CAD build for the part. Positions are in the model's coordinates, mm. Round coordinates to 2 decimals unless told otherwise and drop trailing zeros. Order: outer loops, then holes, each group sorted by start corner. A loop starts at its lowest first (then second) coordinate and runs counter-clockwise, first axis right, second up. Notation, with made-up numbers: (17, 74.5) -> (39, 74.5) arc R19 ccw to (39, 93.5) -> close; hole circle Ø2 at (83.25, 20). An arc over 180 degrees is marked (long way). Return JSON: item names as keys, results as strings. Group by question number.
Q1. Cut at C-C (y = -5). Count the separate pieces of the cut face and the enclosed holes in it, then the cut area to 3 significant figures.
Q2. Cut at A-A (x = 138). Write the cut outline in (y, z).
Q3. Probe line 1 along Z through (x, y) = (354.5, -9.5); line 2 along Z through (x, y) = (149.5, -2.25); line 3 along Z through (x, y) = (480.5, -7.25). List the from-to ranges inside material, lowest first.
Q4. Cut at B-B (z = 173.5). Write the cut outline in (x, y), then the cut area to 3 significant figures.
Q5. Flat gauge pins, fed straight in: pin 1 (5 mm diameter, centred on y = -9, z = 80.5, fed in from +X); pin 2 (5 mm diameter, centred on x = 439, y = -6.5, fed in from +Z). Where does each tip first touch, or does it go through?
Q6. Cut at D-D (x = 213.5). Write the cut outline in (y, z).
from build123d import *

# Parameters (mm, degrees)
PAD_DEPTH       = 10
SKETCH001_W     = 379
SKETCH001_H     = 305
SKETCH001_W_2   = 413
SKETCH001_H_2   = 45
POCKET_DEPTH    = 10.001
SKETCH002_W     = 50
SKETCH002_H     = 10
POCKET001_DEPTH = 10.001


with BuildPart() as part:
    # Sketch → Pad (new body)
    with BuildSketch(Plane.XZ):
        Polygon((0, 0), (560, 0), (570, 0), (570, 50), (560, 50), (560, 212), (570, 212), (570, 262), (560, 262), (560, 424), (570, 424), (570, 474), (560, 474), (0, 474), (-10, 474), (-10, 424), (0, 424), (0, 262), (-10, 262), (-10, 212), (0, 212), (0, 50), (-10, 50), (-10, 0), align=None)
    extrude(amount=PAD_DEPTH)

    # Sketch001 → Pocket (cut, through all)
    with BuildSketch(Plane.XZ.offset(10)):
        with Locations((285, 277.802533)):
            Rectangle(SKETCH001_W, SKETCH001_H)
        with Locations((285, 87.802533)):
            Rectangle(SKETCH001_W_2, SKETCH001_H_2)
    extrude(amount=-POCKET_DEPTH, mode=Mode.SUBTRACT)

    # Sketch002 → Pocket001 (cut, through all)
    with BuildSketch(Plane.XZ.offset(10)):
        with Locations((130, 469)):
            Rectangle(SKETCH002_W, SKETCH002_H)
        with Locations((430, 469)):
            Rectangle(SKETCH002_W, SKETCH002_H)
    extrude(amount=-POCKET001_DEPTH, mode=Mode.SUBTRACT)


solid = part.part
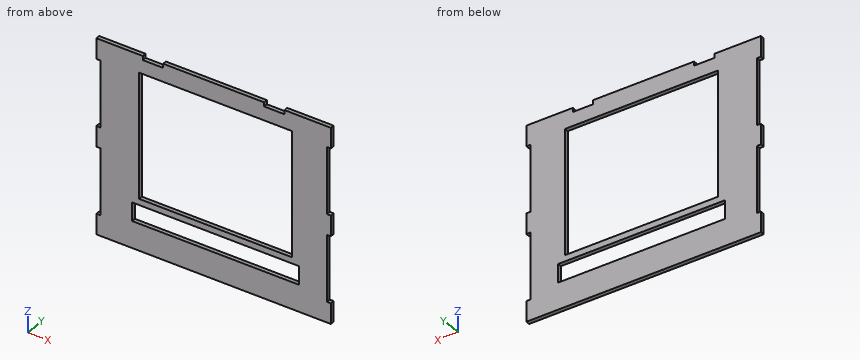
Solution:
{
 "1": {"separate pieces": "1", "enclosed holes": "2", "area": "133,000 mm²"},
 "2": {"outline": "(-10, 0) -> (0, 0) -> (0, 65.3) -> (-10, 65.3) -> close; (-10, 110.3) -> (0, 110.3) -> (0, 125.3) -> (-10, 125.3) -> close; (-10, 430.3) -> (0, 430.3) -> (0, 464) -> (-10, 464) -> close"},
 "3": {"line 1": "z = 0 to 65.3, 110.3 to 125.3, 430.3 to 474", "line 2": "z = 0 to 65.3, 110.3 to 125.3, 430.3 to 464", "line 3": "z = 0 to 65.3, 110.3 to 474"},
 "4": {"outline": "(0, -10) -> (95.5, -10) -> (95.5, 0) -> (0, 0) -> close; (474.5, -10) -> (560, -10) -> (560, 0) -> (474.5, 0) -> close", "area": "1,810 mm²"},
 "5": {"pin 1": "stops at x = 560", "pin 2": "stops at z = 464"},
 "6": {"outline": "(-10, 0) -> (0, 0) -> (0, 65.3) -> (-10, 65.3) -> close; (-10, 110.3) -> (0, 110.3) -> (0, 125.3) -> (-10, 125.3) -> close; (-10, 430.3) -> (0, 430.3) -> (0, 474) -> (-10, 474) -> close"}
}
